Part model, mm, in its own coordinate system. A direction names the side the tool comes from. Round coordinates to 2 decimals unless told otherwise and drop trailing zeros. Order: outer loops, then holes, each group sorted by start corner. A loop starts at its lowest first (then second) coordinate and runs counter-clockwise, first axis right, second up. Notation, with made-up numbers: M 58,76.5 L 93,76.5 A23 ccw 93,93.5 Z; hole C 40,-13 d3. An arc over 180 degrees is marked long. One line per question, with ' | ' between items.
from build123d import *

# Parameters (mm, degrees)
SKETCH1_W           = 40
SKETCH1_H           = 43
BOSS_EXTRUDE1_DEPTH = 19
SKETCH2_W           = 19
SKETCH2_H           = 2.54
BOSS_EXTRUDE2_DEPTH = 7.62
SKETCH3_R           = 1.5
CUT_EXTRUDE1_DEPTH  = 63.292927367
SKETCH4_W           = 19
SKETCH4_H           = 2.54
BOSS_EXTRUDE3_DEPTH = 7.62
SKETCH5_R           = 1.5
CUT_EXTRUDE2_DEPTH  = 63.292927367


with BuildPart() as part:
    # Sketch1 → Boss-Extrude1 (new body)
    with BuildSketch(Plane.XY):
        with Locations((20, 21.5)):
            Rectangle(SKETCH1_W, SKETCH1_H)
    extrude(amount=BOSS_EXTRUDE1_DEPTH)

    # Sketch2 → Boss-Extrude2 (add)
    with BuildSketch(Plane(origin=(40, 0, 0), x_dir=(0, 0, -1), z_dir=(1, 0, 0))):
        with Locations((-9.5, 34.11)):
            Rectangle(SKETCH2_W, SKETCH2_H)
    extrude(amount=BOSS_EXTRUDE2_DEPTH)

    # Sketch3 → Cut-Extrude1 (cut, through all)
    with BuildSketch(Plane(origin=(0, 35.38, 0), x_dir=(1, 0, 0), z_dir=(0, 1, 0))):
        with Locations(Location((45.08, -3.81, 0), (0, 0, 270))):
            Circle(SKETCH3_R)
        with Locations(Location((45.08, -15.19, 0), (0, 0, 270))):
            Circle(SKETCH3_R)
    extrude(amount=-CUT_EXTRUDE1_DEPTH, mode=Mode.SUBTRACT)

    # Sketch4 → Boss-Extrude3 (add)
    with BuildSketch(Plane.ZY):
        with Locations((9.5, 34.11)):
            Rectangle(SKETCH4_W, SKETCH4_H)
    extrude(amount=BOSS_EXTRUDE3_DEPTH)

    # Sketch5 → Cut-Extrude2 (cut, through all)
    with BuildSketch(Plane(origin=(0, 35.38, 0), x_dir=(1, 0, 0), z_dir=(0, 1, 0))):
        with Locations(Location((-5.08, -3.81, 0), (0, 0, 270))):
            Circle(SKETCH5_R)
        with Locations(Location((-5.08, -15.19, 0), (0, 0, 270))):
            Circle(SKETCH5_R)
    extrude(amount=-CUT_EXTRUDE2_DEPTH, mode=Mode.SUBTRACT)


solid = part.part
1) Saw through at C-C (z = 15). List the corners of the cut face in (x, y), plus the area to 3 significant figures.
The answers:
outline: M -7.62,32.84 L -6.57,32.84 L -6.57,35.38 L -7.62,35.38 Z; M -3.59,32.84 L 0,32.84 L 0,0 L 40,0 L 40,32.84 L 43.59,32.84 L 43.59,35.38 L 40,35.38 L 40,43 L 0,43 L 0,35.38 L -3.59,35.38 Z; M 46.57,32.84 L 47.62,32.84 L 47.62,35.38 L 46.57,35.38 Z | area: 1,740 mm²
2) Which spindle directions (+Z, -Z, +X, -X, +Y, -Y) get a long thin tool onto all of the face, cutting with end or side? Do faces 5 (the face through (0, 39, 9)), 6 (the face through (44, 32.84, 10)), 7 (the face through (47.62, 34, 10)), 8 (the face through (40, 39, 9)), 9 (the face through (0, 16, 9)). Say none if no direction does.
The answers:
face 5: +Z, -Z, -X, +Y | face 6: +Z, -Z, +X, -Y | face 7: +Z, -Z, +X, +Y, -Y | face 8: +Z, -Z, +X, +Y | face 9: +Z, -Z, -X, -Y
3) Saw through at A-A (z = 3.81). List the corners of the cut face in (x, y).
The answers:
outline: M -7.62,32.84 L -6.58,32.84 L -6.58,35.38 L -7.62,35.38 Z; M -3.58,32.84 L 0,32.84 L 0,0 L 40,0 L 40,32.84 L 43.58,32.84 L 43.58,35.38 L 40,35.38 L 40,43 L 0,43 L 0,35.38 L -3.58,35.38 Z; M 46.58,32.84 L 47.62,32.84 L 47.62,35.38 L 46.58,35.38 Z
4) Drop flat-ended pins along their axis: pin 1 (2.5 mm diameter, centred on x = -2.5, z = 7.5, fed in from -Y); pin 2 (1 mm diameter, centred on y = 9, z = 11, fed in from -X); pin 3 (4 mm diameter, centred on x = -5, z = 14, fed in from +Y); pin 4 (2.5 mm diameter, centred on x = -5.08, z = 15.19, fed in from -Y). Give the stop position or say it passes through.
The answers:
pin 1: stops at y = 32.84 | pin 2: stops at x = 0 | pin 3: stops at y = 35.38 | pin 4: passes through
5) Saw through at B-B (x = -5.08). List the corners of the cut face in (y, z).
The answers:
outline: M 32.84,0 L 35.38,0 L 35.38,2.31 L 32.84,2.31 Z; M 32.84,5.31 L 35.38,5.31 L 35.38,13.69 L 32.84,13.69 Z; M 32.84,16.69 L 35.38,16.69 L 35.38,19 L 32.84,19 Z
6) Probe line 1 (X direction, y = 34.85, z = 3.81); line 2 (Z direction, x = 45, y = 33); line 3 (X direction, y = 12, z = 11.25). List the from-to ranges inside material, lowest first. Write a range as [from, to].
The answers:
line 1: x = [-7.62, -6.58], [-3.58, 43.58], [46.58, 47.62] | line 2: z = [0, 2.31], [5.31, 13.69], [16.69, 19] | line 3: x = [0, 40]
7) Saw through at D-D (y = 40). List the corners of the cut face in (x, z), plus the area to 3 significant figures.
The answers:
outline: M 0,0 L 40,0 L 40,19 L 0,19 Z | area: 760 mm²
8) Two-plate mould, pull along Z, no slides. Class faces 1 (the face through (20, 22, 19)), 2 (the face through (46.567, 34.128, 3.615)), 3 (the face through (20, 22, 0)), 4 (the face through (44, 35.38, 10)): released by +Z, released by -Z, zero draft, split by the parting line, or undercut.
The answers:
face 1: released by +Z | face 2: undercut | face 3: released by -Z | face 4: zero draft
